Verification items for the finished model (mm, model axes). Face numbers are marked on the shaded views. A direction names the side the tool comes from. Give positions to 0.01 mm unless a question says otherwise; leave off trailing zeros. Loops run counter-clockwise (first coordinate to the right, second up) from the corner with the lowest first, then second, coordinate; pieces in that order, holes last. Notation, with made-up numbers: (16.5, 11) - (48.5, 11) arc R24 cw to (48.5, 34) - close; hole circle Ø2 at (62.5, 82). An arc over 180 degrees is marked (long way). Use one line per item in the form item = value.
```python
from build123d import *

# Parameters (mm, degrees)
SKETCH_1_R          = 2.5
EXTRUDE_1_DEPTH     = 51
CUT_EXTRUDE_START   = -15
CUT_EXTRUDE_1_DEPTH = 15
CHAMFER_1_SIZE      = 0.5


with BuildPart() as part:
    # Эскиз1 → Бобышка-Вытянуть1 (new body)
    with BuildSketch(Plane(origin=(0, 0, 0), x_dir=(1, 0, 0), z_dir=(0, 1, 0))):
        with Locations(Location((0, 0, 0), (0, 0, 270))):
            Circle(SKETCH_1_R)
    extrude(amount=EXTRUDE_1_DEPTH)

    # Эскиз2 → Вырез-Вытянуть1 (cut)
    with BuildSketch(Plane(origin=(0, 51, 0), x_dir=(1, 0, 0), z_dir=(0, 1, 0)).offset(CUT_EXTRUDE_START)):
        with BuildLine():
            Line((-1.5, 2), (1.5, 2))
            ThreePointArc((1.5, 2), (0, 2.5), (-1.5, 2))
        make_face()
    extrude(amount=CUT_EXTRUDE_1_DEPTH, mode=Mode.SUBTRACT)

    # Фаска1
    chamfer_1_edges = [part.edges().sort_by_distance(p)[0] for p in [
        (-2.371708245, 51, 0.790569415),
        (0, 0, -2.5),
    ]]
    chamfer(chamfer_1_edges, length=CHAMFER_1_SIZE - 0.0001)  # a hair under: the kernel refuses the full size


solid = part.part
```
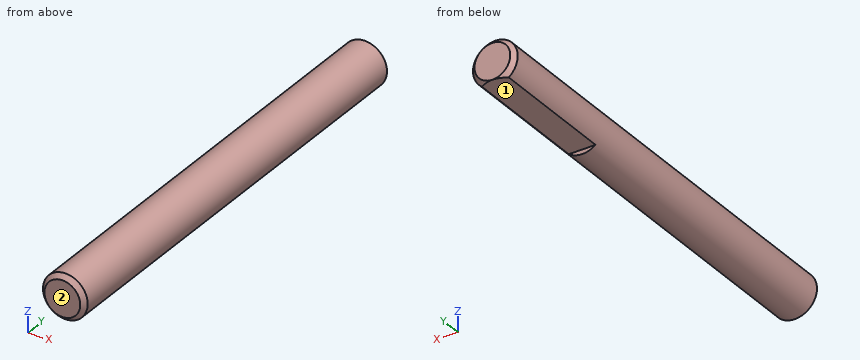
1. Tool access check on the marked faces 1 and 2. Record the directions out of +Z, -Z, +X, -X, +Y, -Y that give a thin tool (end or side, any length) a straight path to the whole face; none if there is none.
Result set:
face_1 = -Z, +X, -X, +Y
face_2 = +Z, -Z, +X, -X, -Y
2. Scan lines: probe 1 along X at (y, z) = (31.5, -0.1); probe 2 along Z at (x, y) = (0.2, 8.5); probe 3 along Z at (x, y) = (1.15, 38). Record each from-to range of solid material in increasing order.
Result set:
probe_1 = -2.5 to 2.5
probe_2 = -2.49 to 2.49
probe_3 = -2 to 2.22
3. Depth check by flat-ended pin: pin 1 Ø1 at (y, z) = (37, 1) entering from +X. Enter the tip coordinate at first touch or a pass-through.
Result set:
pin_1 = 2.45
4. Section check A-A, the plane y = 16.5. Record the cut outline in (x, z), then the cut area to 3 significant figures.
Result set:
outline = circle Ø5 at (0, 0)
area = 19.6 mm²
